Design review of the part built by this model. Coordinates are the model's own, in mm. A direction names the side the tool comes from. Round coordinates to 2 decimals unless told otherwise and drop trailing zeros. Loops run counter-clockwise (first coordinate to the right, second up) from the corner with the lowest first, then second, coordinate; pieces in that order, holes last. Notation, with made-up numbers: M -17,-24.5 L -1,-24.5 A20 ccw -1,7.5 Z; hole C 48.25,-23 d6. An arc over 180 degrees is marked long. One line per item, written item: value. Start each with the question number.
Item 1: Clearance check with flat-ended pins moving along their axes: pin 1 (2.5 mm diameter, centred on x = 15.5, z = -15.5, fed in from +Y); pin 2 (5 mm diameter, centred on x = 15.5, z = 3.5, fed in from +Y); pin 3 (3.5 mm diameter, centred on x = -15.5, z = -15.5, fed in from -Y); pin 4 (10 mm diameter, centred on x = -16.5, z = 4, fed in from +Y). State where each tip first meets the part, or that it passes through.
Item 2: Mouldability with a two-part tool opening along Y and no side actions: class faces 4 (the flat face through (3, 28.5, 0)), 5 (the flat face through (0, 41.5, 0)), 6 (the flat face through (19.2, -0.3, 19.1)) as released by +Y, released by -Y, zero draft, split by the parting line, or undercut.
Item 3: For line 1 along Z through (x, y) = (15.5, -1); line 2 along Z through (x, y) = (-15, 0), list the stretches that pass through material, from the lowest coordinate up.
Item 4: For faces 1 (the flat face through (-2, 40.5, -6)), 2 (the cylindrical face through (-1.73, 41.01, 7.81)), 3 (the flat face through (-19.1, -0.3, 19.2)), list the 3-axis set-ups (+Z, -Z, +X, -X, +Y, -Y) from which the entire face can be reached by the end or side of a thin tool; tool diameter is ignored.
Item 5: We need section B-B (y = -5.5). Write out the cut boundary in (x, z).
Item 6: We need section D-D (x = -10). Write out the cut boundary in (y, z).
Item 7: We need section C-C (z = 0). Write out the cut boundary in (x, y), then the cut area to 3 significant figures.
Item 8: We need section A-A (x = -15.5). Write out the cut boundary in (y, z).
from build123d import *

# Parameters (mm, degrees)
CROQUIS1_W              = 42.3
CROQUIS1_H              = 42.3
CROQUIS1_R              = 1.5
SALIENTE_EXTRUIR1_DEPTH = 19.5
CROQUIS2_R              = 12.5
SALIENTE_EXTRUIR2_DEPTH = 2
CROQUIS3_R              = 2.5
SALIENTE_EXTRUIR3_DEPTH = 20
CROQUIS4_R              = 8
SALIENTE_EXTRUIR4_DEPTH = 1
CROQUIS5_R              = 6
SALIENTE_EXTRUIR5_DEPTH = 12
CHAFL_N1_SIZE           = 4


with BuildPart() as part:
    # Croquis1 → Saliente-Extruir1 (new body, symmetric)
    with BuildSketch(Plane(origin=(0, 0, 0), x_dir=(1, 0, 0), z_dir=(0, 1, 0))):
        Rectangle(CROQUIS1_W, CROQUIS1_H)
        with Locations((15.5, 15.5)):
            Circle(CROQUIS1_R, mode=Mode.SUBTRACT)
        with Locations((15.5, -15.5)):
            Circle(CROQUIS1_R, mode=Mode.SUBTRACT)
        with Locations((-15.5, -15.5)):
            Circle(CROQUIS1_R, mode=Mode.SUBTRACT)
        with Locations((-15.5, 15.5)):
            Circle(CROQUIS1_R, mode=Mode.SUBTRACT)
    extrude(amount=SALIENTE_EXTRUIR1_DEPTH, both=True)

    # Croquis2 → Saliente-Extruir2 (add)
    with BuildSketch(Plane(origin=(0, 19.5, 0), x_dir=(1, 0, 0), z_dir=(0, 1, 0))):
        Circle(CROQUIS2_R)
    extrude(amount=SALIENTE_EXTRUIR2_DEPTH)

    # Croquis3 → Saliente-Extruir3 (add)
    with BuildSketch(Plane(origin=(0, 21.5, 0), x_dir=(1, 0, 0), z_dir=(0, 1, 0))):
        Circle(CROQUIS3_R)
    extrude(amount=SALIENTE_EXTRUIR3_DEPTH)

    # Croquis4 → Saliente-Extruir4 (add)
    with BuildSketch(Plane(origin=(0, 41.5, 0), x_dir=(1, 0, 0), z_dir=(0, 1, 0))):
        Circle(CROQUIS4_R)
    extrude(amount=-SALIENTE_EXTRUIR4_DEPTH)

    # Croquis5 → Saliente-Extruir5 (add)
    with BuildSketch(Plane.XZ.offset(-40.5)):
        Circle(CROQUIS5_R)
    extrude(amount=SALIENTE_EXTRUIR5_DEPTH)

    # Chaflán1
    chafl_n1_edges = [part.edges().sort_by_distance(p)[0] for p in [
        (21.15, 0, 21.15),
        (-21.15, 0, 21.15),
        (-21.15, 0, -21.15),
        (21.15, 0, -21.15),
    ]]
    chamfer(chafl_n1_edges, length=CHAFL_N1_SIZE)


solid = part.part
A:
1. pin 1: through
1. pin 2: y = 19.5
1. pin 3: y = -19.5
1. pin 4: y = 21.5
2. face 4: undercut
2. face 5: released by +Y
2. face 6: zero draft
3. line 1: -21.15 to -17, -14 to 14, 17 to 21.15
3. line 2: -21.15 to -16.91, -14.09 to 14.09, 16.91 to 21.15
4. face 1: none
4. face 2: +Y
4. face 3: +Z, -X, +Y, -Y
5. outline: M -21.15,-17.15 L -17.15,-21.15 L 17.15,-21.15 L 21.15,-17.15 L 21.15,17.15 L 17.15,21.15 L -17.15,21.15 L -21.15,17.15 Z; hole C -15.5,-15.5 d3; hole C -15.5,15.5 d3; hole C 15.5,-15.5 d3; hole C 15.5,15.5 d3
6. outline: M -19.5,-21.15 L 19.5,-21.15 L 19.5,-7.5 L 21.5,-7.5 L 21.5,7.5 L 19.5,7.5 L 19.5,21.15 L -19.5,21.15 Z
7. outline: M -21.15,-19.5 L 21.15,-19.5 L 21.15,19.5 L 12.5,19.5 L 12.5,21.5 L 2.5,21.5 L 2.5,28.5 L 6,28.5 L 6,40.5 L 8,40.5 L 8,41.5 L -8,41.5 L -8,40.5 L -6,40.5 L -6,28.5 L -2.5,28.5 L -2.5,21.5 L -12.5,21.5 L -12.5,19.5 L -21.15,19.5 Z
7. area: 1,890 mm2
8. outline: M -19.5,-21.15 L 19.5,-21.15 L 19.5,-17 L -19.5,-17 Z; M -19.5,-14 L 19.5,-14 L 19.5,14 L -19.5,14 Z; M -19.5,17 L 19.5,17 L 19.5,21.15 L -19.5,21.15 Z
